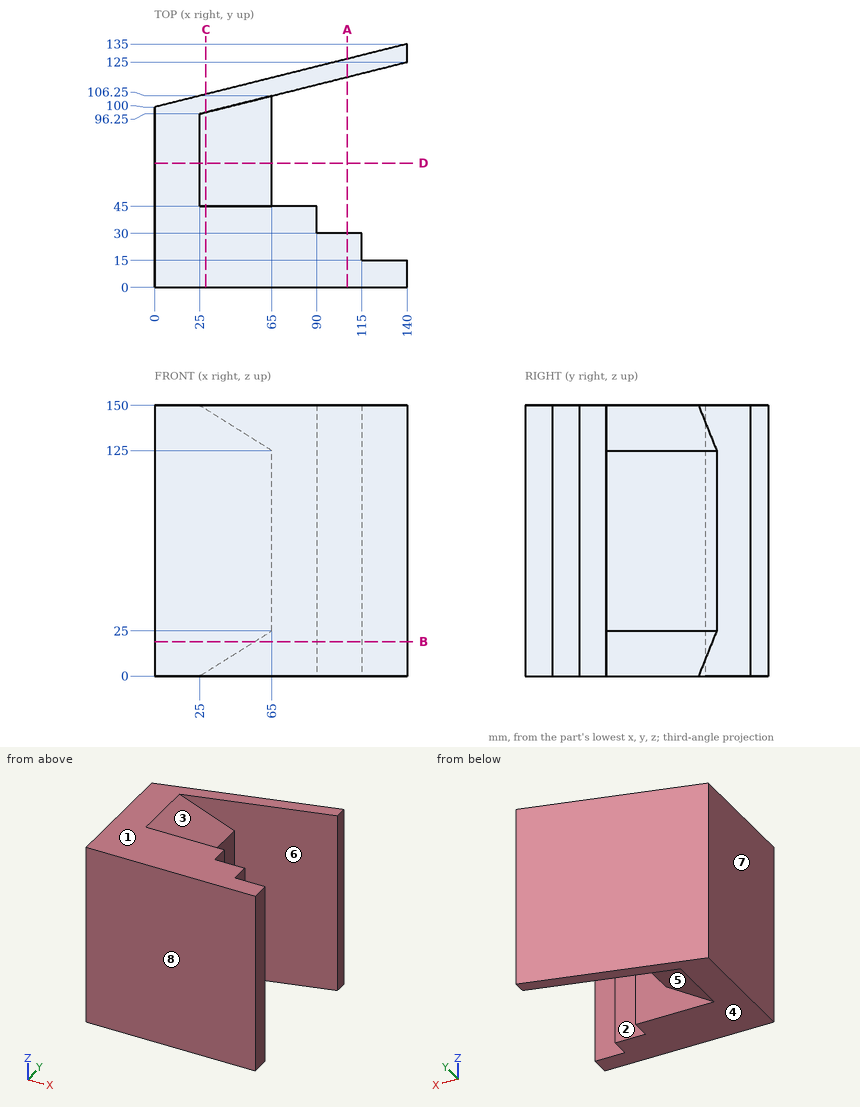
Verification items for this drawing (mm, ordinates from the low corner). A direction names the side the tool comes from. Coordinates: 2 decimals unless noted, no trailing zeros. Loops run counter-clockwise (first coordinate to the right, second up) from the corner with the lowest first, then second, coordinate; pieces in that order, holes last. Notation, with made-up numbers: (26, -20.5) -> (39, -20.5) arc R21 ccw to (39, -1.5) -> close; hole circle Ø9 at (37.25, -13.75). An arc over 180 degrees is marked (long way). Answer in a Markdown table with one row per item. Add a question column.
1. Section check C-C, the plane x = 28.5. Enter the section's corners in (y, z) (1 decimal).
2. Draft check along Y on the marked faces 6, 7 and 8. Enter one of: +Y half, -Y half, draft (parallel to the pull), parting line (faces both ways), or undercut.
3. Depth check by flat-ended pin: P1, Ø4, axis at x = 73.5, y = 109, coming from the -Z side; P2, Ø6, axis at x = 42, y = 54, coming from the -Z side; P3, Ø3, axis at x = 71.5, z = 71, coming from the +Y side; P4, Ø7.5, axis at x = 123.5, z = 39, coming from the +Y side. Enter the tip coordinate at first touch or a pass-through.
4. Access from +Z, -Z, +X, -X, +Y, -Y to the whole of each face (thin tool, end or side, straight path). Record for the marked faces 1, 2, 3, 4 and 5.
5. Section check D-D, the plane y = 69. Enter the section's corners in (x, z).
6. Section check B-B, the plane z = 19. Enter the section's corners in (x, y), then the cut area to 3 significant figures.
7. Material ranges on probe 1 along Y at (x, z) = (118.5, 16) (3 decimals); probe 2 along Y at (x, z) = (124, 62.5); probe 3 along X at (y, z) = (28.5, 107.5), recorded low to high. Write a range as [from, to].
8. Section check A-A, the plane x = 107. Enter the section's corners in (y, z), then the cut area to 3 significant figures.
Derived:
| question | item | result |
|---|---|---|
| 1 | outline | (0, 0) -> (45, 0) -> (45, 2.2) -> (97.1, 2.2) -> (97.1, 0) -> (107.1, 0) -> (107.1, 150) -> (97.1, 150) -> (97.1, 147.8) -> (45, 147.8) -> (45, 150) -> (0, 150) -> close |
| 2 | face 6 | undercut |
| 2 | face 7 | draft |
| 2 | face 8 | -Y half |
| 3 | P1 | stops at z = 0 |
| 3 | P2 | stops at z = 8.75 |
| 3 | P3 | stops at y = 118.25 |
| 3 | P4 | stops at y = 131.81 |
| 4 | face 1 | +Z, +X, -X, +Y, -Y |
| 4 | face 2 | +Z, -Z, +X |
| 4 | face 3 | +Z, +X |
| 4 | face 4 | -Z, +X, -X, +Y, -Y |
| 4 | face 5 | -Z, +X |
| 5 | outline | (0, 0) -> (25, 0) -> (65, 25) -> (65, 125) -> (25, 150) -> (0, 150) -> close |
| 6 | outline | (0, 0) -> (140, 0) -> (140, 15) -> (115, 15) -> (115, 30) -> (90, 30) -> (90, 45) -> (55.4, 45) -> (55.4, 103.85) -> (140, 125) -> (140, 135) -> (0, 100) -> close |
| 6 | area | 9,450 mm² |
| 7 | probe 1 | y = [0, 15], [119.625, 129.625] |
| 7 | probe 2 | y = [0, 15], [121, 131] |
| 7 | probe 3 | x = [0, 115] |
| 8 | outline | (0, 0) -> (30, 0) -> (30, 150) -> (0, 150) -> close; (116.75, 0) -> (126.75, 0) -> (126.75, 150) -> (116.75, 150) -> close |
| 8 | area | 6,000 mm² |
